Read the model definition and answer for the solid it produces. Units are mm, in the model's axes. Face numbers are marked on the shaded views. A direction names the side the tool comes from. Coordinates: 2 decimals unless noted, no trailing zeros. Order: outer loops, then holes, each group sorted by start corner. A loop starts at its lowest first (then second) coordinate and runs counter-clockwise, first axis right, second up. Notation, with made-up numbers: (5, -27.75) -> (46, -27.75) arc R23 ccw to (46, -18.75) -> close; hole circle Ø8 at (-24, 72.5). An arc over 180 degrees is marked (long way). Answer in a Markdown table with one row per item.
Autodesk Inventor part; units mm, degrees
ref_plane "YZ Plane" through (0, 0, 0) normal (1, 0, 0) x (0, 1, 0)
ref_plane "XZ Plane" through (0, 0, 0) normal (0, 1, 0) x (-1, 0, 0)
ref_plane "XY Plane" through (0, 0, 0) normal (0, 0, 1) x (1, 0, 0)
sketch "Sketch1" plane through (0, 0, 0) normal (0, 0, 1) x (1, 0, 0)
  line L0 (-50, 50) -> (50, 50)
  line L1 (50, 50) -> (50, -50)
  line L2 (50, -50) -> (-50, -50)
  line L3 (-50, -50) -> (-50, 50)
  line L4 (0, 0) -> (0, 7.629) construction
  line L5 (0, 0) -> (6.8797, 0) construction
  dimension "d0" = 100
  dimension "d1" = 100
extrude "Extrusion1" add sketch "Sketch1" along normal blind 20
sketch "Sketch2" plane through (50, -50, 0) normal (1, 0, 0) x (0, 0, -1)
  line L0 (-20, 100) -> (-20, 0)
  line L1 (-20, 15) -> (-10, 9.2265)
  line L2 (-10, 9.2265) -> (-10, 90.7735)
  line L3 (-10, 90.7735) -> (-20, 85)
  line L4 (0, 0) -> (-20, 0)
  line L5 (0, 100) -> (-20, 100)
  point P0 (0, 50)
  dimension "d4" = 60
  dimension "d5" = 60
  dimension "d6" = 10
  dimension "d7" = 15
  dimension "d8" = 15
extrude "Extrusion2" cut sketch "Sketch2" against normal blind 118.25
sketch "Sketch3" plane through (-50, -50, 0) normal (0, -1, 0) x (1, 0, 0)
  line L0 (100, 10) -> (0, 10)
  line L1 (0, 0) -> (0, 20)
  line L2 (0, 20) -> (100, 20)
  line L3 (100, 0) -> (100, 20)
  point P0 (50, 0)
  point P1 (25, 14)
  point P2 (75, 14)
  dimension "d11" = 25
  dimension "d12" = 6
  dimension "d21" = 25
hole "Hole1" at (-25, -50, 14) at (25, -50, 14) direction (0, 1, 0) diameter 3.242 end through all
sketch "Sketch4" plane through (-50, -50, 0) normal (0, -1, 0) x (1, 0, 0)
  circle A0 centre (5, 5) radius 1.6
  circle A1 centre (14, 5) radius 1.6
  point P0 (50, 0)
hole "Hole2" at (-45, -50, 5) at (-36, -50, 5) direction (0, 1, 0) diameter 2.459 depth 9 tip angle 118
properties part number "3d_LM-Welding_Tooling - Fixed base" material "Aluminium 6061-T6"
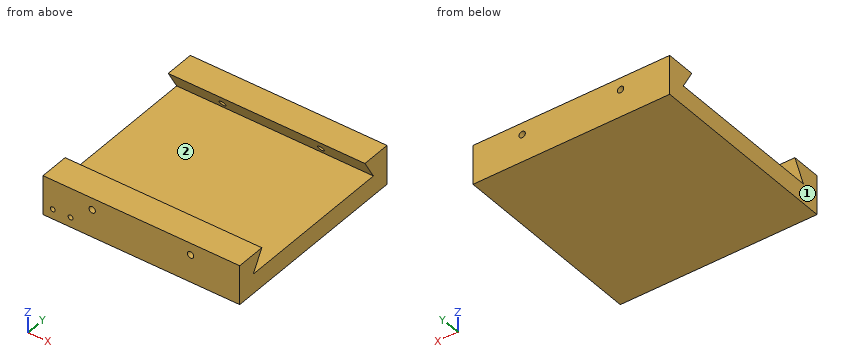
Q1. The part is cut by section B-B (z = 17.25). Write down the section's boundary in (x, y), then the cut area to 3 significant figures.
Outcome:
| item | result |
|---|---|
| outline | (-50, -50) -> (50, -50) -> (50, -36.59) -> (-50, -36.59) -> close; (-50, 36.59) -> (50, 36.59) -> (50, 50) -> (-50, 50) -> close |
| area | 2,680 mm² |
Q2. The part is cut by section C-C (x = -25). Write down the section's boundary in (y, z), then the cut area to 3 significant figures.
Outcome:
| item | result |
|---|---|
| outline | (-50, 0) -> (50, 0) -> (50, 12.38) -> (39.4, 12.38) -> (40.77, 10) -> (-40.77, 10) -> (-39.4, 12.38) -> (-50, 12.38) -> close; (-50, 15.62) -> (-37.53, 15.62) -> (-35, 20) -> (-50, 20) -> close; (35, 20) -> (37.53, 15.62) -> (50, 15.62) -> (50, 20) -> close |
| area | 1,170 mm² |
Q3. Given pin 1 (10 mm diameter, centred on x = -35, y = 16, fed in from +Z); pin 2 (1.5 mm diameter, centred on x = -45, z = 5, fed in from -Y), each flat-ended and moving along its own axis, determine where each tip first touches the part or whether it passes through.
Outcome:
| item | result |
|---|---|
| pin 1 | z = 10 |
| pin 2 | y = -40.71 |
Q4. Consider line 1 (X direction, y = 42.25, z = 14); line 2 (Z direction, x = -25, y = 42); line 3 (Z direction, x = -0.5, y = -30). Determine where each line is inside the solid, lowest interval first.
Outcome:
| item | result |
|---|---|
| line 1 | -50 to -26.62, -23.38 to 23.38, 26.62 to 50 |
| line 2 | 0 to 12.38, 15.62 to 20 |
| line 3 | 0 to 10 |
Q5. For the marked faces 1 and 2, determine the directions among +Z, -Z, +X, -X, +Y, -Y from which every point of the face is accessible in a straight line to the end or side of a thin tool.
Outcome:
| item | result |
|---|---|
| face 1 | +Z, -Z, -X, +Y, -Y |
| face 2 | +X, -X |
Q6. The part is cut by section D-D (y = -20.5). Write down the section's boundary in (x, z), then the cut area to 3 significant figures.
Outcome:
| item | result |
|---|---|
| outline | (-50, 0) -> (50, 0) -> (50, 10) -> (-50, 10) -> close |
| area | 1,000 mm² |
Q7. The part is cut by section A-A (x = 3). Write down the section's boundary in (y, z), then the cut area to 3 significant figures.
Outcome:
| item | result |
|---|---|
| outline | (-50, 0) -> (50, 0) -> (50, 20) -> (35, 20) -> (40.77, 10) -> (-40.77, 10) -> (-35, 20) -> (-50, 20) -> close |
| area | 1,240 mm² |
